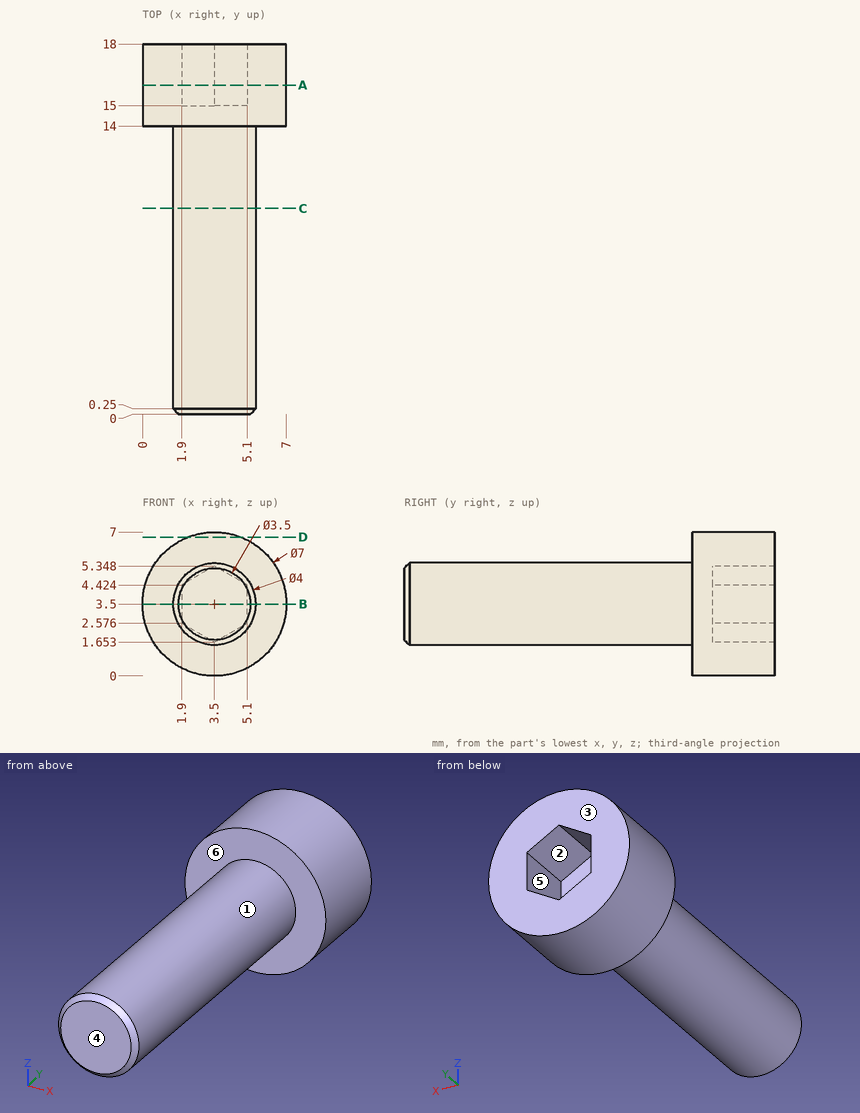
Design review of the part shown in the three views and the two pictorial views. Dimensions are in mm from the part's minimum x, y and z. A direction names the side the tool comes from. Give positions to 0.01 mm unless a question says otherwise; leave off trailing zeros. Loops run counter-clockwise (first coordinate to the right, second up) from the corner with the lowest first, then second, coordinate; pieces in that order, holes last. Notation, with made-up numbers: M -33,72.5 L 15,72.5 A19 ccw 15,76.5 Z; hole C 75,-7 d5. An arc over 180 degrees is marked long. Answer as a JSON object with one key per item and string values. Group by question number.
Q1. Add section A-A on y = 16. Give the boundary of the cut face in (x, z).
Q2. Add section B-B on z = 3.5. Give the boundary of the cut face in (x, y).
Q3. Add section D-D on z = 6.75. Give the boundary of the cut face in (x, y).
Q4. For probe 1 along X at (y, z) = (16.5, 3.5); probe 2 along Y at (x, z) = (2.5, 5.5); probe 3 along Z at (x, y) = (3.5, 8), list the stretches that pass through material, from the lowest coordinate up. Write a range as [from, to].
Q5. Mouldability with a two-part tool opening along X and no side actions: class the marked faces 1, 2 and 3 as +X half, -X half, draft (parallel to the pull), parting line (faces both ways), or undercut.
Q6. Add section C-C on y = 10. Give the boundary of the cut face in (x, z), and give its area (3 significant figures).
Q7. Tool access review of the marked faces 4, 5 and 6: name each direction out of +Z, -Z, +X, -X, +Y, -Y from which nothing blocks a thin tool from reaching the whole face with its end or side.
Q8. Insertion check: P1, Ø0.6, axis at y = 16.5, z = 4, coming from the -X side; P2, Ø2, axis at x = 5, y = 3.5, coming from the -Z side; P3, Ø0.9, axis at y = 16.5, z = 3, coming from the +X side; P4, Ø4, axis at x = 1.5, y = 11.5, coming from the +Z side. Each pin has a flat end and moves straight along its axis. Give the tip position at first contact, or say it passes through.
Checked values:
{
 "1": {"outline": "C 3.5,3.5 d7; hole M 1.9,2.58 L 3.5,1.65 L 5.1,2.58 L 5.1,4.42 L 3.5,5.35 L 1.9,4.42 Z"},
 "2": {"outline": "M 0,14 L 1.5,14 L 1.5,0.25 L 1.75,0 L 5.25,0 L 5.5,0.25 L 5.5,14 L 7,14 L 7,18 L 5.1,18 L 5.1,15 L 1.9,15 L 1.9,18 L 0,18 Z"},
 "3": {"outline": "M 2.2,14 L 4.8,14 L 4.8,18 L 2.2,18 Z"},
 "4": {"probe 1": "[0, 1.9], [5.1, 7]", "probe 2": "[14, 18]", "probe 3": "[1.5, 5.5]"},
 "5": {"face 1": "parting line", "face 2": "undercut", "face 3": "draft"},
 "6": {"outline": "C 3.5,3.5 d4", "area": "12.6 mm²"},
 "7": {"face 4": "+Z, -Z, +X, -X, -Y", "face 5": "+Y", "face 6": "-Y"},
 "8": {"P1": "x = 0.01", "P2": "z = 1.56", "P3": "x = 7", "P4": "z = 5.5"}
}
